```python
from build123d import *

# Parameters (mm, degrees)
F1_DEPTH  = 90
F3_DEPTH  = 10
F5_DEPTH  = 90
F6_SIZE   = 1
F8_DEPTH  = 8
F9_R      = 3.25
F10_DEPTH = 25
F12_DEPTH = 25
F11_W     = 31.5
F11_H     = 13.2
F13_DEPTH = 1.25
F14_R     = 5
F14_R_2   = 3
F15_DEPTH = 6
F16_DEPTH = 25


with BuildPart() as f1:
    # F0 (on Front) → F1 (new body)
    with BuildSketch(Plane.XZ):
        Polygon((5, 131), (0, 131), (0, 0), (5, 0), (5, 19), (11, 19), (11, 15), (15, 15), (15, 117), (11, 117), (11, 113), (5, 113), align=None)
        Polygon((5, 0), (0, 0), (0, -5.121096503), (87, -5.121096503), (87, 0), align=None)
    extrude(amount=F1_DEPTH)

    # F2 (on face) → F3 (join)
    with BuildSketch(Plane.XZ.offset(90)):
        Polygon((87, -5.121096503), (87, 0), (5, 0), (5, 19), (11, 19), (11, 15), (15, 15), (15, 117), (11, 117), (11, 113), (5, 113), (5, 131), (0, 131), (0, -5.121096503), align=None)
        Polygon((5, 0), (87, 0), (87, 12), (17, 131), (5, 131), (5, 113), (11, 113), (11, 117), (15, 117), (15, 15), (11, 15), (11, 19), (5, 19), align=None)
    extrude(amount=F3_DEPTH)

    # F4 (on face) → F5 (cut)
    with BuildSketch(Plane(origin=(0, 0, 0), x_dir=(0, -1, 0), z_dir=(-1, 0, 0))):
        Polygon((100, 131), (94, 131), (100, 11.878903497), align=None)
    extrude(amount=-F5_DEPTH, mode=Mode.SUBTRACT)

    # F6
    f6_edges = [f1.edges().sort_by_distance(p)[0] for p in [
        (8, 0, 113),
        (11, 0, 115),
        (13, 0, 117),
        (15, 0, 66),
        (13, 0, 15),
        (11, 0, 17),
        (8, 0, 19),
    ]]
    chamfer(f6_edges, length=F6_SIZE)

    # F7 (on face) → F8 (cut)
    with BuildSketch(Plane(origin=(0, -90, 0), x_dir=(-1, 0, 0), z_dir=(0, 1, 0))):
        Polygon((-25.625, 1.125), (-25.625, 11.625), (-44.025, 11.625), (-47.025, 9.075), (-47.025, 3.675), (-44.025, 1.125), align=None)
    extrude(amount=-F8_DEPTH, mode=Mode.SUBTRACT)

    # F9 (on face) → F10 (cut)
    with BuildSketch(Plane(origin=(0, -98, 0), x_dir=(-1, 0, 0), z_dir=(0, 1, 0))):
        with Locations((-41.825, 6.375)):
            Circle(F9_R)
        with Locations((-30.825, 6.375)):
            Circle(F9_R)
    extrude(amount=-F10_DEPTH, mode=Mode.SUBTRACT)

    # F11 (on face) → F12 (cut)
    with BuildSketch(Plane.XZ.offset(90)):
        with BuildLine():
            ThreePointArc((58.6058854217, 1.6786588252), (58.9474129273, 1.0847088218), (59.5910971765, 0.85))
            Line((59.5910971765, 0.85), (74.9089028235, 0.85))
            ThreePointArc((74.9089028235, 0.85), (75.5525870727, 1.0847088218), (75.8941145783, 1.6786588252))
            Line((75.8941145783, 1.6786588252), (77.5462884913, 11.1786588252))
            ThreePointArc((77.5462884913, 11.1786588252), (77.3263679147, 11.9936842492), (76.5610767365, 12.35))
            Line((76.5610767365, 12.35), (57.9389232635, 12.35))
            ThreePointArc((57.9389232635, 12.35), (57.1736320853, 11.9936842492), (56.9537115087, 11.1786588252))
            Line((56.9537115087, 11.1786588252), (58.6058854217, 1.6786588252))
        make_face()
    extrude(amount=F12_DEPTH, mode=Mode.SUBTRACT)

    # F11 (on face) → F13 (cut)
    with BuildSketch(Plane.XZ.offset(90)):
        with Locations((67.25, 6.6)):
            Rectangle(F11_W, F11_H)
        with BuildLine():
            Line((74.9089028235, 0.85), (59.5910971765, 0.85))
            ThreePointArc((59.5910971765, 0.85), (58.9474129273, 1.0847088218), (58.6058854217, 1.6786588252))
            Line((58.6058854217, 1.6786588252), (56.9537115087, 11.1786588252))
            ThreePointArc((56.9537115087, 11.1786588252), (57.1736320853, 11.9936842492), (57.9389232635, 12.35))
            Line((57.9389232635, 12.35), (76.5610767365, 12.35))
            ThreePointArc((76.5610767365, 12.35), (77.3263679147, 11.9936842492), (77.5462884913, 11.1786588252))
            Line((77.5462884913, 11.1786588252), (75.8941145783, 1.6786588252))
            ThreePointArc((75.8941145783, 1.6786588252), (75.5525870727, 1.0847088218), (74.9089028235, 0.85))
        make_face(mode=Mode.SUBTRACT)
    extrude(amount=F13_DEPTH, mode=Mode.SUBTRACT)

    # F14 (on face) → F15 (cut)
    with BuildSketch(Plane.YZ.offset(15)):
        with Locations((-45.5, 97)):
            Circle(F14_R)
        with Locations((-45.5, 97)):
            Circle(F14_R_2, mode=Mode.SUBTRACT)
        with Locations((-45.5, 35)):
            Circle(F14_R)
        with Locations((-45.5, 35)):
            Circle(F14_R_2, mode=Mode.SUBTRACT)
    extrude(amount=-F15_DEPTH, mode=Mode.SUBTRACT)

    # F16 (cut): faces of the model
    f16_faces = [f1.faces().sort_by_distance(p)[0] for p in [
        (15, -45.5, 97),
        (15, -45.5, 35),
    ]]
    extrude(f16_faces, amount=-F16_DEPTH, mode=Mode.SUBTRACT)


solid = f1.part
```
Verification items for the finished model (mm, model axes). A direction names the side the tool comes from. Give positions to 0.01 mm unless a question says otherwise; leave off trailing zeros. Order: outer loops, then holes, each group sorted by start corner. A loop starts at its lowest first (then second) coordinate and runs counter-clockwise, first axis right, second up. Notation, with made-up numbers: (88.5, 33) - (112.5, 33) arc R21 cw to (112.5, 45) - close; hole circle Ø1 at (-40, 88). An arc over 180 degrees is marked (long way). Answer as CSV lines item,"result". Start each with the question number.
Item 1: Section check C-C, the plane z = 46. Record the boundary of the cut face in (x, y), plus the area to 3 significant figures.
Item 2: Gauge pin test, flat ends, axial feed: pin 1 (5 mm diameter, centred on y = -45.5, z = 97, fed in from +X); pin 2 (5 mm diameter, centred on x = 9, y = -25.5, fed in from +Z); pin 3 (10 mm diameter, centred on x = 20, z = 102, fed in from -Y); pin 4 (10 mm diameter, centred on y = -31.5, z = 84.5, fed in from +X). Record the tip position at first contact, or that the pin passes through.
Item 3: Mould release check, pull along Z, two halves, no side actions. Record for faces 4 (the face through (60.27, -93.82, 57.44)), 5 (the face through (15, -45, 65)), 6 (the face through (45.5, -93.94, 10.37)): released by +Z, released by -Z, zero draft, split by the parting line, or undercut.
Item 4: Material ranges on L1, parallel to Z at x = 7, y = -45.5; L2, parallel to Z at x = 12.2, y = -45.5; L3, parallel to Z at x = 2.5, y = -45.5, recorded low to high.
Item 5: Section check B-B, the plane z = 97. Record the boundary of the cut face in (x, y).
Item 6: Section check A-A, the plane y = -45.5. State how many separate pieces and enclosed holes the cut face has, plus the area to 3 significant figures.
Item 7: Access from +Z, -Z, +X, -X, +Y, -Y to the whole of each face (thin tool, end or side, straight path). Record for faces 1 (the face through (12, -49.5, 94)), 2 (the face through (13, -45, 15)), 3 (the face through (67, -91.25, 13)).
Filled in:
1,outline,"(0, -98.28) - (67, -98.28) - (67, -90) - (15, -90) - (15, -1) - (14, 0) - (0, 0) - close"
1,area,"1,900 mm^2"
2,pin 1,"through"
2,pin 2,"z = 117"
2,pin 3,"y = -95.71"
2,pin 4,"x = 15"
3,face 4,"released by +Z"
3,face 5,"zero draft"
3,face 6,"undercut"
4,L1,"-5.12 to 0, 19 to 32, 38 to 94, 100 to 113"
4,L2,"-5.12 to 0, 15 to 30, 40 to 92, 102 to 117"
4,L3,"-5.12 to 32, 38 to 94, 100 to 131"
5,outline,"(0, -95.71) - (37, -95.71) - (37, -90) - (15, -90) - (15, -50.5) - (9, -50.5) - (9, -48.5) - (0, -48.5) - close; (0, -42.5) - (9, -42.5) - (9, -40.5) - (15, -40.5) - (15, -1) - (14, 0) - (0, 0) - close"
6,separate pieces,"3"
6,enclosed holes,"0"
6,area,"1,840 mm^2"
7,face 1,"+X"
7,face 2,"+X, +Y"
7,face 3,"+Y"
